Geometry: final body of the model. Coordinates: model frame, mm. A direction names the side the tool comes from. Give positions to 0.01 mm unless a question says otherwise; leave off trailing zeros. Write each loop counter-clockwise with the first axis right and the second up, starting at its lowest first coordinate (ties: lowest second). Pieces come first, ordered by that corner, then holes. Notation, with made-up numbers: (58, 60) -> (102, 60) arc R21 ccw to (102, 89) -> close; hole circle Ø3 at (10, -18.75). An arc over 180 degrees is marked (long way). Answer as a JSON object with one key per item and string values. Group by question number.
(1) Section query C-C on x = 31.5. Output: boundary loops of the cut face in (y, z), plus the area to 3 significant figures.
(2) Material intervals for probe 1 along Y at (x, z) = (0.5, 204.5) (3 decimals); probe 2 along X at (y, z) = (10, 211.75); probe 3 along Z at (x, y) = (20, -31), sorted ascending.
(3) Section query D-D on y = -20. Output: boundary loops of the cut face in (x, z).
(4) Set-up query: faces 1 (the face through (-39, -30, 195)), 2 (the face through (25, -14, 25)), 3 (the face through (-18.74, -8.45, 215.07)), 4 (the face through (-0.33, 19.33, 112.48)), 5 (the face through (-1, -38, 25)). Return all of +Z, -Z, +X, -X, +Y, -Y with unobstructed straight access to the full face (end or side cutting, diameter ignored); none if empty.
(5) Contact query for flat-ended pins moving along their axis: pin 1 Ø4 at (x, y) = (-17.32, 10) entering from -Z; pin 2 Ø1.5 at (x, z) = (-13, 147) entering from +Y; pin 3 Ø8 at (x, z) = (-38, 201.5) entering from +Y; pin 4 Ø9 at (x, z) = (45, 25) entering from +Y. Output: stop coordinate, or through.
(6) Section query A-A on z = 25. Output: boundary loops of the cut face in (x, y), plus the area to 3 significant figures.
(7) Draft query along X for faces 6 (the face through (1.863, 19.031, 213.098)), 7 (the face through (15.46, 10.97, 6.9)), 8 (the face through (0, -32, 210)), 9 (the face through (25, -14, 195)). Return one class per face: +X half, -X half, draft (parallel to the pull), parting line (faces both ways), or undercut.
(8) Section query B-B on x = 45. Output: boundary loops of the cut face in (y, z).
from build123d import *

# Parameters (mm, degrees)
SKETCH1_R                 = 25
SKETCH1_R_2               = 15
BOSS_EXTRUDE1_DEPTH       = 220
CIRPATTERN1_COUNT         = 6
SKETCH11_R                = 7.5
CUT_EXTRUDE2_DEPTH        = 1
SKETCH13_W                = 120
SKETCH13_H                = 30
BOSS_EXTRUDE3_DEPTH       = 38
SKETCH15_R                = 15
CUT_EXTRUDE3_DEPTH        = 221.0000001
SKETCH16_W                = 35
SKETCH16_H                = 30
CUT_EXTRUDE4_DEPTH        = 38
MIRROR4_COPY_1_SKETCH_W   = 35
MIRROR4_COPY_1_SKETCH_H   = 30
MIRROR4_COPY_1_DEPTH      = 38
FILLET1_R                 = 5
FILLET2_R                 = 3
M6X1_0_TAPPED_HOLE1_D     = 5
M6X1_0_TAPPED_HOLE1_DEPTH = 17
M6X1_0_TAPPED_HOLE1_TIP   = 1.502151548
LPATTERN1_COUNT           = 2
LPATTERN1_PITCH           = 90
LPATTERN1_COUNT_DIR2      = 2
LPATTERN1_PITCH_DIR2      = 170


with BuildPart() as part:
    # Sketch1 → Boss-Extrude1 (new body)
    with BuildSketch(Plane.XY):
        Circle(SKETCH1_R)
        Circle(SKETCH1_R_2, mode=Mode.SUBTRACT)
    extrude(amount=BOSS_EXTRUDE1_DEPTH)

    # Sketch2 → M5x0.8 Tapped Hole1 (revolve, cut)
    with BuildSketch(Plane(origin=(0, 20, 220), x_dir=(0, -1, 0), z_dir=(1, 0, 0))):
        Polygon((0, 0), (0, 15.2618073), (2.1, 14), (2.1, 0), align=None)
    m5x0_8_tapped_hole1 = revolve(axis=Axis((0, 20, 226.35), (0, 0, -1)), mode=Mode.SUBTRACT)

    # CirPattern1: M5x0.8 Tapped Hole1 ×6 about axis
    cirpattern1_axis = Axis((0, 0, 0), (0, 0, 1))
    for i in range(1, CIRPATTERN1_COUNT):
        add(m5x0_8_tapped_hole1.rotate(cirpattern1_axis, i * 360 / CIRPATTERN1_COUNT), mode=Mode.SUBTRACT)

    # Mirror1: M5x0.8 Tapped Hole1 across plane
    add(m5x0_8_tapped_hole1.mirror(Plane.XY.offset(110)), mode=Mode.SUBTRACT)

    # Mirror1 copy 1 sketch → Mirror1 copy 1 (revolve, cut)
    with BuildSketch(Plane(origin=(-17.320508076, 10, 0), x_dir=(0.866025404, -0.5, 0), z_dir=(0.5, 0.866025404, 0))):
        Polygon((0, 0), (0, -15.2618073), (2.1, -14), (2.1, 0), align=None)
    revolve(axis=Axis((-17.320508076, 10, -6.35), (0, 0, -1)), mode=Mode.SUBTRACT)

    # Mirror1 copy 2 sketch → Mirror1 copy 2 (revolve, cut)
    with BuildSketch(Plane(origin=(-17.320508076, -10, 0), x_dir=(0.866025404, 0.5, 0), z_dir=(-0.5, 0.866025404, 0))):
        Polygon((0, 0), (0, -15.2618073), (2.1, -14), (2.1, 0), align=None)
    revolve(axis=Axis((-17.320508076, -10, -6.35), (0, 0, -1)), mode=Mode.SUBTRACT)

    # Mirror1 copy 3 sketch → Mirror1 copy 3 (revolve, cut)
    with BuildSketch(Plane(origin=(0, -20, 0), x_dir=(0, 1, 0), z_dir=(-1, 0, 0))):
        Polygon((0, 0), (0, -15.2618073), (2.1, -14), (2.1, 0), align=None)
    revolve(axis=Axis((0, -20, -6.35), (0, 0, -1)), mode=Mode.SUBTRACT)

    # Mirror1 copy 4 sketch → Mirror1 copy 4 (revolve, cut)
    with BuildSketch(Plane(origin=(17.320508076, -10, 0), x_dir=(-0.866025404, 0.5, 0), z_dir=(-0.5, -0.866025404, 0))):
        Polygon((0, 0), (0, -15.2618073), (2.1, -14), (2.1, 0), align=None)
    revolve(axis=Axis((17.320508076, -10, -6.35), (0, 0, -1)), mode=Mode.SUBTRACT)

    # Mirror1 copy 5 sketch → Mirror1 copy 5 (revolve, cut)
    with BuildSketch(Plane(origin=(17.320508076, 10, 0), x_dir=(-0.866025404, -0.5, 0), z_dir=(0.5, -0.866025404, 0))):
        Polygon((0, 0), (0, -15.2618073), (2.1, -14), (2.1, 0), align=None)
    revolve(axis=Axis((17.320508076, 10, -6.35), (0, 0, -1)), mode=Mode.SUBTRACT)

    # Sketch11 → Cut-Extrude2 (cut)
    with BuildSketch(Plane(origin=(0, 25, 0), x_dir=(-1, 0, 0), z_dir=(0, 1, 0))):
        with Locations((0, 110)):
            Circle(SKETCH11_R)
    extrude(amount=-CUT_EXTRUDE2_DEPTH, mode=Mode.SUBTRACT)

    # Sketch13 → Boss-Extrude3 (add)
    with BuildSketch(Plane(origin=(0, 0, 0), x_dir=(1, 0, 0), z_dir=(0, 1, 0))):
        with Locations((0, -195)):
            Rectangle(SKETCH13_W, SKETCH13_H)
    boss_extrude3 = extrude(amount=-BOSS_EXTRUDE3_DEPTH)

    # Mirror2: Boss-Extrude3 across plane
    add(boss_extrude3.mirror(Plane.XY.offset(110)))

    # Sketch15 → Cut-Extrude3 (cut, through all)
    with BuildSketch(Plane.XY.offset(220)):
        Circle(SKETCH15_R)
    extrude(amount=-CUT_EXTRUDE3_DEPTH, mode=Mode.SUBTRACT)

    # Sketch16 → Cut-Extrude4 (cut)
    with BuildSketch(Plane.XY.offset(210)):
        with Locations((-42.5, -15)):
            Rectangle(SKETCH16_W, SKETCH16_H)
    cut_extrude4 = extrude(amount=-CUT_EXTRUDE4_DEPTH, mode=Mode.SUBTRACT)

    # Mirror3: Cut-Extrude4 across plane
    add(cut_extrude4.mirror(Plane(origin=(0, 0, 0), x_dir=(0, 0, 1), z_dir=(1, 0, 0))), mode=Mode.SUBTRACT)

    # Mirror4: Cut-Extrude4 across plane
    add(cut_extrude4.mirror(Plane.XY.offset(110)), mode=Mode.SUBTRACT)

    # Mirror4 copy 1 sketch → Mirror4 copy 1 (cut)
    with BuildSketch(Plane(origin=(0, 0, 10), x_dir=(-1, 0, 0), z_dir=(0, 0, -1))):
        with Locations((-42.5, -15)):
            Rectangle(MIRROR4_COPY_1_SKETCH_W, MIRROR4_COPY_1_SKETCH_H)
    extrude(amount=-MIRROR4_COPY_1_DEPTH, mode=Mode.SUBTRACT)

    # Fillet1
    fillet1_edges = [part.edges().sort_by_distance(p)[0] for p in [
        (-60, -30, 195),
        (60, -30, 195),
        (60, -30, 25),
        (-60, -30, 25),
    ]]
    fillet(fillet1_edges, radius=FILLET1_R)

    # Fillet2
    fillet2_edges = [part.edges().sort_by_distance(p)[0] for p in [
        (-25, -30, 195),
        (25, -30, 195),
        (25, -30, 25),
        (-25, -30, 25),
    ]]
    fillet(fillet2_edges, radius=FILLET2_R)

    # Sketch19 → Ø10.0 (10) Diameter Hole1 (revolve, cut)
    with BuildSketch(Plane(origin=(-45, -30, 25), x_dir=(0, 0, 1), z_dir=(1, 0, 0))):
        Polygon((0, 0), (0, 14.004303095), (5, 11), (5, 0), align=None)
    f_10_0_10_diameter_hole1 = revolve(axis=Axis((-45, -23.65, 25), (0, -1, 0)), mode=Mode.SUBTRACT)

    # M6x1.0 Tapped Hole1
    with Locations(Plane(origin=(0, 24, 0), x_dir=(-1, 0, 0), z_dir=(0, 1, 0))):
        with Locations((0, 110)):
            Hole(M6X1_0_TAPPED_HOLE1_D / 2, depth=M6X1_0_TAPPED_HOLE1_DEPTH)
            with Locations((0, 0, -(M6X1_0_TAPPED_HOLE1_DEPTH + M6X1_0_TAPPED_HOLE1_TIP / 2))):  # 118° drill point
                Cone(0, M6X1_0_TAPPED_HOLE1_D / 2, M6X1_0_TAPPED_HOLE1_TIP, mode=Mode.SUBTRACT)

    # LPattern1: 10.0 _10_ Diameter Hole1 2 × 2
    with Locations(*[(i * LPATTERN1_PITCH, 0, j * LPATTERN1_PITCH_DIR2) for i in range(LPATTERN1_COUNT) for j in range(LPATTERN1_COUNT_DIR2) if (i, j) != (0, 0)]):
        add(f_10_0_10_diameter_hole1, mode=Mode.SUBTRACT)


solid = part.part
Answer list:
{
 "1": {"outline": "(-38, 10) -> (-30, 10) -> (-30, 40) -> (-38, 40) -> close; (-38, 180) -> (-30, 180) -> (-30, 210) -> (-38, 210) -> close", "area": "480 mm2"},
 "2": {"probe 1": "-38 to -14.992, 14.992 to 24.995", "probe 2": "-22.91 to -19.42, -15.22 to -11.18, 11.18 to 15.22, 19.42 to 22.91", "probe 3": "10 to 40, 180 to 210"},
 "3": {"outline": "(-25, 10) -> (-15, 10) -> (-15, 0) -> (-2.1, 0) -> (-2.1, 10) -> (2.1, 10) -> (2.1, 0) -> (15, 0) -> (15, 10) -> (25, 10) -> (25, 40) -> (15, 40) -> (15, 180) -> (25, 180) -> (25, 210) -> (15, 210) -> (15, 220) -> (2.1, 220) -> (2.1, 210) -> (-2.1, 210) -> (-2.1, 220) -> (-15, 220) -> (-15, 210) -> (-25, 210) -> (-25, 180) -> (-15, 180) -> (-15, 40) -> (-25, 40) -> close"},
 "4": {"face 1": "+Z, -Z, -X, +Y", "face 2": "+Z, -Z, +X, +Y", "face 3": "+Z", "face 4": "+Y", "face 5": "+Z, -Z, +X, -X, -Y"},
 "5": {"pin 1": "z = 14.06", "pin 2": "y = 21.79", "pin 3": "y = -30", "pin 4": "through"},
 "6": {"outline": "(-60, -38) -> (-50, -38) -> (-50, -30) -> (-55, -30) arc R5 ccw to (-60, -35) -> close; (-40, -38) -> (40, -38) -> (40, -30) -> (28, -30) arc R3 cw to (25, -27) -> (25, 0) arc R25 ccw to (-25, 0) -> (-25, -27) arc R3 cw to (-28, -30) -> (-40, -30) -> close; (50, -38) -> (60, -38) -> (60, -35) arc R5 ccw to (55, -30) -> (50, -30) -> close; hole circle Ø30 at (0, 0)", "area": "2,570 mm2"},
 "7": {"face 6": "undercut", "face 7": "undercut", "face 8": "draft", "face 9": "+X half"},
 "8": {"outline": "(-38, 10) -> (-30, 10) -> (-30, 20) -> (-38, 20) -> close; (-38, 30) -> (-30, 30) -> (-30, 40) -> (-38, 40) -> close; (-38, 180) -> (-30, 180) -> (-30, 190) -> (-38, 190) -> close; (-38, 200) -> (-30, 200) -> (-30, 210) -> (-38, 210) -> close"}
}
